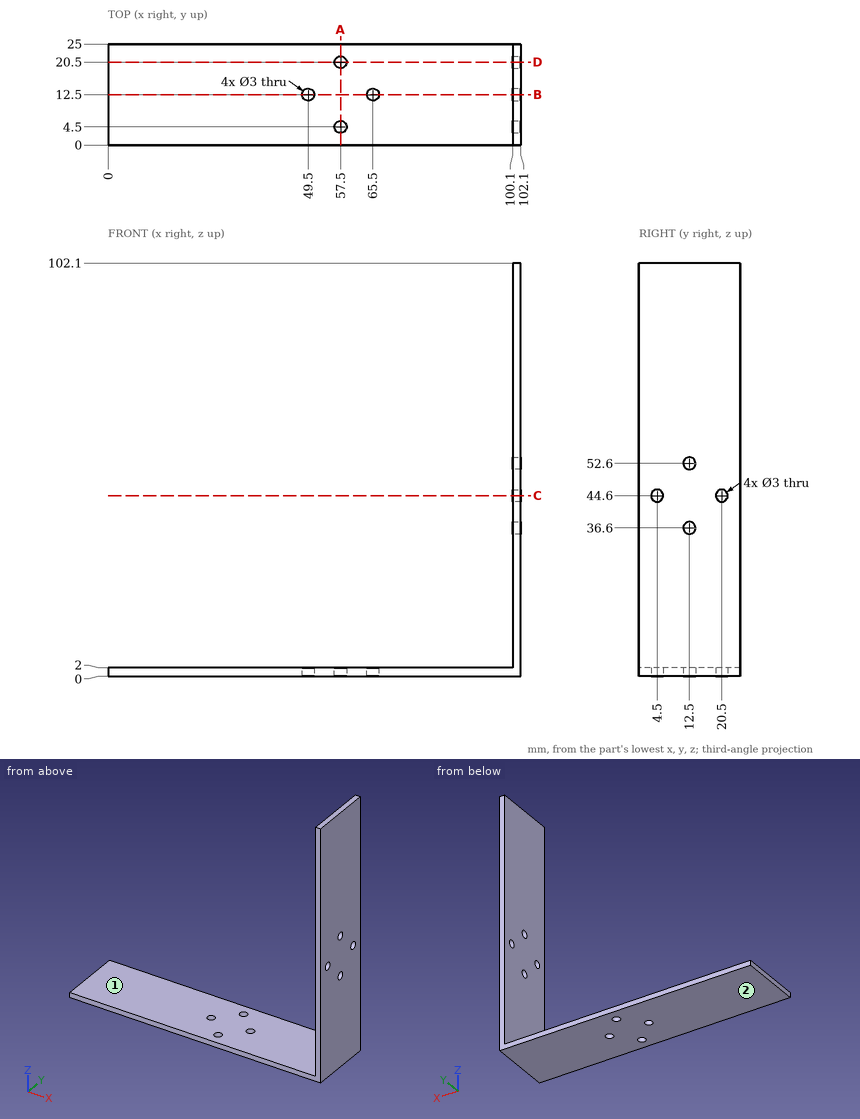
Source: three-view drawing plus pictorial views. Frame: mm from the lowest corner of the part. A direction names the side the tool comes from. Round coordinates to 2 decimals unless told otherwise and drop trailing zeros. Order: outer loops, then holes, each group sorted by start corner. A loop starts at its lowest first (then second) coordinate and runs counter-clockwise, first axis right, second up. Notation, with made-up numbers: (-4, 38) -> (25, 38) arc R21 ccw to (25, 51) -> close; hole circle Ø2 at (-24.5, 20.25). An arc over 180 degrees is marked (long way). Use one line per item in the form item = value. Start each with the question number.
1. Cut plane D-D (y = 20.5). Return the cut outline in (x, z), then the cut area to 3 significant figures.
2. Line query: probe 1 along Y at (x, z) = (101.55, 44.6); probe 2 along Z at (x, y) = (101.4, 4.5); probe 3 along Y at (x, z) = (65.5, 1.55). Output: solid intervals per line, ascending.
3. Cut plane A-A (x = 57.5). Return the cut outline in (y, z).
4. Cut plane C-C (z = 44.6). Return the cut outline in (x, y).
5. Reachability of the marked faces 1 and 2 from +Z, -Z, +X, -X, +Y, -Y: full face, straight path, thin tool, end or side. Return the list, or none.
6. Pin query (flat end, axial travel): pin 1 Ø1.8 at (x, y) = (49.5, 12.5) entering from -Z; pin 2 Ø3 at (y, z) = (16, 41) entering from -X; pin 3 Ø3 at (x, y) = (80, 13.5) entering from +Z. Return the tip coordinate at first contact, or that it passes through.
7. Cut plane B-B (y = 12.5). Return the cut outline in (x, z), then the cut area to 3 significant figures.
Solution:
q1.outline = (0, 0) -> (56, 0) -> (56, 2) -> (0, 2) -> close; (59, 0) -> (102.1, 0) -> (102.1, 43.1) -> (100.1, 43.1) -> (100.1, 2) -> (59, 2) -> close; (100.1, 46.1) -> (102.1, 46.1) -> (102.1, 102.1) -> (100.1, 102.1) -> close
q1.area = 392 mm^2
q2.probe_1 = 0 to 3, 6 to 19, 22 to 25
q2.probe_2 = 0 to 43.1, 46.1 to 102.1
q2.probe_3 = 0 to 11, 14 to 25
q3.outline = (0, 0) -> (3, 0) -> (3, 2) -> (0, 2) -> close; (6, 0) -> (19, 0) -> (19, 2) -> (6, 2) -> close; (22, 0) -> (25, 0) -> (25, 2) -> (22, 2) -> close
q4.outline = (100.1, 0) -> (102.1, 0) -> (102.1, 3) -> (100.1, 3) -> close; (100.1, 6) -> (102.1, 6) -> (102.1, 19) -> (100.1, 19) -> close; (100.1, 22) -> (102.1, 22) -> (102.1, 25) -> (100.1, 25) -> close
q5.face_1 = +Z, -X, +Y, -Y
q5.face_2 = -Z, +X, -X, +Y, -Y
q6.pin_1 = through
q6.pin_2 = 100.1
q6.pin_3 = 2
q7.outline = (0, 0) -> (48, 0) -> (48, 2) -> (0, 2) -> close; (51, 0) -> (64, 0) -> (64, 2) -> (51, 2) -> close; (67, 0) -> (102.1, 0) -> (102.1, 35.1) -> (100.1, 35.1) -> (100.1, 2) -> (67, 2) -> close; (100.1, 38.1) -> (102.1, 38.1) -> (102.1, 51.1) -> (100.1, 51.1) -> close; (100.1, 54.1) -> (102.1, 54.1) -> (102.1, 102.1) -> (100.1, 102.1) -> close
q7.area = 380 mm^2
